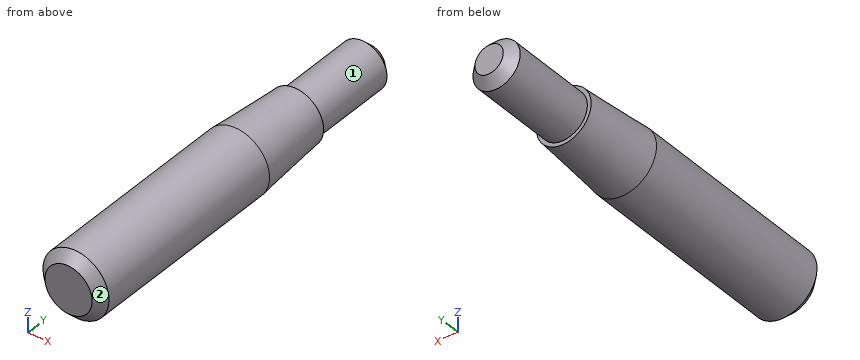
from build123d import *

# Parameters (mm, degrees)
SKETCH2_R           = 7
BOSS_EXTRUDE1_DEPTH = 45
SKETCH3_R           = 7
BOSS_EXTRUDE2_DEPTH = 16
BOSS_EXTRUDE2_TAPER = 4.289
SKETCH4_R           = 5
BOSS_EXTRUDE3_DEPTH = 20
CHAMFER1_SIZE       = 2


with BuildPart() as part:
    # Sketch2 → Boss-Extrude1 (new body)
    with BuildSketch(Plane(origin=(0, 0, 0), x_dir=(1, 0, 0), z_dir=(0, 1, 0))):
        with Locations(Location((0, 0, 0), (0, 0, 90))):
            Circle(SKETCH2_R)
    extrude(amount=BOSS_EXTRUDE1_DEPTH)

    # Sketch3 → Boss-Extrude2 (add)
    with BuildSketch(Plane(origin=(0, 45, 0), x_dir=(1, 0, 0), z_dir=(0, 1, 0))):
        with Locations(Location((0, 0, 0), (0, 0, 90))):
            Circle(SKETCH3_R)
    extrude(amount=BOSS_EXTRUDE2_DEPTH, taper=BOSS_EXTRUDE2_TAPER)

    # Sketch4 → Boss-Extrude3 (add)
    with BuildSketch(Plane(origin=(0, 61, 0), x_dir=(1, 0, 0), z_dir=(0, 1, 0))):
        with Locations(Location((0, 0, 0), (0, 0, 270))):
            Circle(SKETCH4_R)
    extrude(amount=BOSS_EXTRUDE3_DEPTH)

    # Chamfer1
    chamfer1_edges = [part.edges().sort_by_distance(p)[0] for p in [
        (0, 0, 7),
        (0, 81, -5),
    ]]
    chamfer(chamfer1_edges, length=CHAMFER1_SIZE)


solid = part.part
Here's how the part is built. I have some questions about the finished solid (model axes, mm). Face numbers are marked on the shaded views. A direction names the side the tool comes from. Coordinates: 2 decimals unless noted, no trailing zeros. Order: outer loops, then holes, each group sorted by start corner. A loop starts at its lowest first (then second) coordinate and runs counter-clockwise, first axis right, second up.
Item 1: If we section it at A-A on z = 0: List the corners of the cut face in (x, y) for me, plus the area to 3 significant figures.
Result sheet:
outline: (-7, 2) - (-5, 0) - (5, 0) - (7, 2) - (7, 45) - (5.8, 61) - (5, 61) - (5, 79) - (3, 81) - (-3, 81) - (-5, 79) - (-5, 61) - (-5.8, 61) - (-7, 45) - close
area: 1,030 mm2
Item 2: For P1, Ø5, axis at x = -4.5, y = 57.5, coming from the -Z side; P2, Ø1, axis at x = -3, z = 3.5, coming from the +Y side; P3, Ø1.5, axis at x = -4, z = -3, coming from the +Y side; P4, Ø6, axis at y = 22.5, z = -2.5, coming from the -X side, each with a flat end and sliding along its axis, tell me the tip position at first contact or that it passes through.
Result sheet:
P1: stops at z = -5.75
P2: stops at y = 79.89
P3: stops at y = 79.75
P4: stops at x = -7
Item 3: I need wall thicknesses on line 1 (X direction, y = 64, z = -4); line 2 (Z direction, x = 5, y = 43); line 3 (X direction, y = 18, z = 5.5). Which ranges of each line are inside material? Lowest first, please.
Result sheet:
line 1: x = -3 to 3
line 2: z = -4.9 to 4.9
line 3: x = -4.33 to 4.33
Item 4: If we section it at B-B on y = 8: List the corners of the cut face in (x, z) for me, plus the area to 3 significant figures.
Result sheet:
outline: circle Ø14 at (0, 0)
area: 154 mm2
Item 5: For the marked faces 1 and 2, which set-ups out of +Z, -Z, +X, -X, +Y, -Y let a thin tool reach every point of the face, with its end or its side?
Result sheet:
face 1: +Y
face 2: -Y
